Read the model definition and answer for the solid it produces. Units are mm, in the model's axes. Round coordinates to 2 decimals unless told otherwise and drop trailing zeros. Order: outer loops, then holes, each group sorted by start corner. A loop starts at its lowest first (then second) coordinate and runs counter-clockwise, first axis right, second up. Notation, with made-up numbers: (63, 71.5) -> (98, 71.5) arc R17 cw to (98, 78.5) -> close; hole circle Ø4 at (61.25, -10). An arc over 180 degrees is marked (long way). Answer as a JSON object with one key per item and string values. Group by question number.
Item 1: Section A-A, the plane y = 6.9 is taken. Write down the section's boundary in (x, z).
Item 2: Section B-B, the plane x = 7.15 is taken. Write down the section's boundary in (y, z).
Item 3: Given P1, Ø1.2, axis at x = 7.15, y = 6.9, coming from the +Z side; P2, Ø2.5, axis at x = 45, z = 1.5, coming from the +Y side, each flat-ended and moving along its own axis, determine where each tip first touches the part or whether it passes through.
Item 4: Consider probe 1 along Y at (x, z) = (7.15, 4.1); probe 2 along Y at (x, z) = (7.15, 1.55); probe 3 along X at (y, z) = (71.05, 1.25). Determine where each line is inside the solid, lowest interval first. Write a range as from..to.
Item 5: Section D-D, the plane x = 27 is taken. Write down the section's boundary in (y, z), plus the area to 4 significant figures.
Item 6: Section C-C, the plane x = 51.15 is taken. Write down the section's boundary in (y, z).
Autodesk Inventor part; units mm, degrees
ref_plane "YZ Plane" through (0, 0, 0) normal (1, 0, 0) x (0, 1, 0)
ref_plane "XZ Plane" through (0, 0, 0) normal (0, 1, 0) x (-1, 0, 0)
ref_plane "XY Plane" through (0, 0, 0) normal (0, 0, 1) x (1, 0, 0)
sketch "Sketch1" plane through (0, 0, 0) normal (0, 0, 1) x (1, 0, 0)
  line L0 (0, 0) -> (71.43, 0)
  line L1 (71.43, 0) -> (71.43, 86.5)
  line L2 (71.43, 86.5) -> (0, 86.5)
  line L3 (0, 86.5) -> (0, 0)
  line L4 (14, 86.5) -> (57.43, 86.5)
  circle A0 centre (6.25, 81.5) radius 1.5
  circle A1 centre (65.18, 81.5) radius 1.5
  line L5 (11.5, 78.5) -> (59.93, 78.5)
  line L6 (59.93, 78.5) -> (59.93, 86.5)
  line L7 (59.93, 86.5) -> (11.5, 86.5)
  line L8 (11.5, 86.5) -> (11.5, 78.5)
  line L9 (11.5, 78.5) -> (59.93, 86.5) construction
  line L10 (59.93, 78.5) -> (11.5, 86.5) construction
  line L11 (35.715, 86.5) -> (35.715, 82.5) construction
  line L12 (2.95, 2.05) -> (68.45, 2.05)
  line L13 (68.45, 2.05) -> (68.45, 76.45)
  line L14 (68.45, 76.45) -> (2.95, 76.45)
  line L15 (2.95, 76.45) -> (2.95, 2.05)
  line L16 (2.95, 2.05) -> (68.45, 76.45) construction
  line L17 (68.45, 2.05) -> (2.95, 76.45) construction
  circle A2 centre (7.15, 72.25) radius 4
  circle A3 centre (51.15, 71.05) radius 4
  circle A4 centre (7.15, 6.9) radius 4
  circle A5 centre (57.45, 12.05) radius 4
  circle A6 centre (7.15, 72.25) radius 1
  circle A7 centre (51.15, 71.05) radius 1
  circle A8 centre (7.15, 6.9) radius 1
  circle A9 centre (57.45, 12.05) radius 1
  line L18 (50.15, 74.923) -> (50.15, 67.177)
  point P0 (11.5, 86.5)
  point P1 (35.7, 39.25)
  point P2 (35.715, 0)
  point P3 (35.7, 2.05)
  point P4 (9.1397, 10.37)
  point P5 (9.1397, 3.43)
  point P6 (8.15, 10.773)
  point P7 (8.15, 3.027)
  dimension "d0" = 71.43
  dimension "d1" = 86.5
  dimension "d8" = 3
  dimension "d9" = 6.25
  dimension "d10" = 5
  dimension "d11" = 3
  dimension "d12" = 5
  dimension "d13" = 6.25
  dimension "d15" = 48.43
  dimension "d16" = 8
  dimension "d17" = 4
  dimension "d19" = 65.5
  dimension "d20" = 74.4
  dimension "d21" = 2.05
  dimension "d22" = 2.95
  dimension "d23" = 4.2
  dimension "d24" = 4.2
  dimension "d25" = 8
  dimension "d26" = 8
  dimension "d27" = 5.4
  dimension "d29" = 4.85
  dimension "d30" = 4.2
  dimension "d31" = 8
  dimension "d34" = 8
  dimension "d35" = 11
  dimension "d36" = 10
  dimension "d37" = 2
  dimension "d38" = 2
  dimension "d39" = 2
  dimension "d40" = 2
  dimension "d55" = 44
extrude "Extrusion1" add sketch "Sketch1" along normal blind 3 contours L3 L2 L8 L5 L6 L1 L0 | A0 | A1 | L15 L14 L13 L12 | A2 | A7 | A3 L18 | L18 A3 | A4 | A5 | A6 | A8 | A9
extrude "Extrusion2" add sketch "Sketch1" along normal blind 6 contours A2 | A7 | A3 L18 | A4 | A5 | A6 | A8 | A9 picked at (54.1155, 70.7487)
hole "Hole2" at (51.15, 71.05, 0) at (7.15, 72.25, 0) at (7.15, 6.9, 0) direction (0, 0, 1) diameter 2 end through all
equation "\"d13\" = d9"
properties part number "Component_shield_layered_PCB_platform"
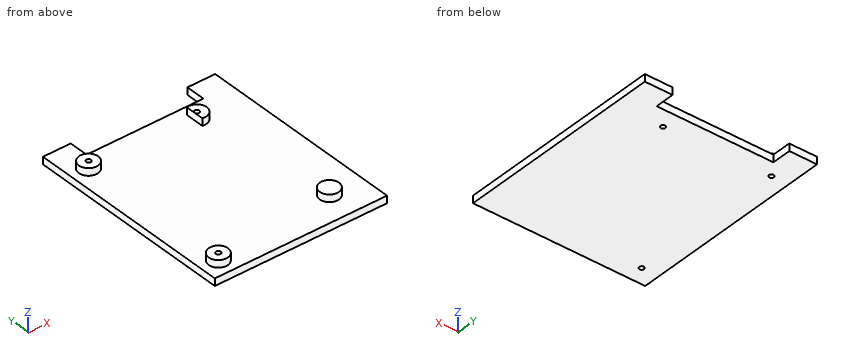
Values found:
{
 "1": {"outline": "(0, 0) -> (6.15, 0) -> (6.15, 6) -> (3.15, 6) -> (3.15, 3) -> (0, 3) -> close; (8.15, 0) -> (71.43, 0) -> (71.43, 3) -> (11.15, 3) -> (11.15, 6) -> (8.15, 6) -> close"},
 "2": {"outline": "(0, 0) -> (5.9, 0) -> (5.9, 6) -> (2.9, 6) -> (2.9, 3) -> (0, 3) -> close; (7.9, 0) -> (71.25, 0) -> (71.25, 6) -> (68.25, 6) -> (68.25, 3) -> (10.9, 3) -> (10.9, 6) -> (7.9, 6) -> close; (73.25, 0) -> (86.5, 0) -> (86.5, 3) -> (76.25, 3) -> (76.25, 6) -> (73.25, 6) -> close"},
 "3": {"P1": "through", "P2": "y = 78.5"},
 "4": {"probe 1": "2.9..5.9, 7.9..10.9, 68.25..71.25, 73.25..76.25", "probe 2": "0..5.9, 7.9..71.25, 73.25..86.5", "probe 3": "0..50.15, 52.15..71.43"},
 "5": {"outline": "(0, 0) -> (78.5, 0) -> (78.5, 3) -> (0, 3) -> close", "area": "235.5 mm2"},
 "6": {"outline": "(0, 0) -> (70.05, 0) -> (70.05, 6) -> (67.05, 6) -> (67.05, 3) -> (0, 3) -> close; (72.05, 0) -> (78.5, 0) -> (78.5, 3) -> (75.05, 3) -> (75.05, 6) -> (72.05, 6) -> close"}
}
